Read the model definition and answer for the solid it produces. Units are mm, in the model's axes. A direction names the side the tool comes from. Round coordinates to 2 decimals unless told otherwise and drop trailing zeros. Order: outer loops, then holes, each group sorted by start corner. A loop starts at its lowest first (then second) coordinate and runs counter-clockwise, first axis right, second up.
Autodesk Inventor part; units mm, degrees
ref_plane "YZ Plane" through (0, 0, 0) normal (1, 0, 0) x (0, 1, 0)
ref_plane "XZ Plane" through (0, 0, 0) normal (0, 1, 0) x (-1, 0, 0)
ref_plane "XY Plane" through (0, 0, 0) normal (0, 0, 1) x (1, 0, 0)
sketch "Sketch1" plane through (0, 0, 0) normal (0, 1, 0) x (-1, 0, 0)
  line L0 (-30, -30) -> (30, -30)
  line L1 (30, -30) -> (30, 30)
  line L2 (30, 30) -> (-30, 30)
  line L3 (-30, 30) -> (-30, -30)
  line L4 (-30, -30) -> (30, 30) construction
  line L5 (30, -30) -> (-30, 30) construction
  circle A0 centre (0, 0) radius 7.5
  circle A1 centre (-25, 25) radius 1.95
  circle A2 centre (0, 25) radius 1.95
  circle A3 centre (0, 25) radius 1.95
  circle A4 centre (25, 0) radius 1.95
  circle A5 centre (25, -25) radius 1.95
  circle A6 centre (-25, 25) radius 1.95
  circle A7 centre (-25, -25) radius 1.95
  circle A8 centre (25, 25) radius 1.95
  circle A9 centre (-25, 0) radius 1.95
  circle A10 centre (0, -25) radius 1.95
  line L6 (28, 30) -> (30, 28)
  line L7 (30, 28) -> (30, -28)
  line L8 (30, -28) -> (28, -30)
  line L9 (28, -30) -> (-28, -30)
  line L10 (-28, -30) -> (-30, -28)
  line L11 (-30, -28) -> (-30, 28)
  line L12 (-30, 28) -> (-28, 30)
  line L13 (-28, 30) -> (28, 30)
  dimension "d0" = 60
  dimension "d1" = 60
  dimension "d13" = 15
extrude "Extrusion1" add sketch "Sketch1" along normal blind 12 contours L3 L10 L0 | L10 L3 L12 L2 L6 L1 L8 L0 | L8 L1 L0 | L3 L2 L12 | L6 L2 L1 | A1 | A2 | A4 | A5 | A7 | A8 | A9 | A10
sketch "Sketch2" plane through (0, 12, 0) normal (0, 1, 0) x (1, 0, 0)
  line L0 (30, 30) -> (-30, 30)
  line L1 (-30, 30) -> (-30, -30)
  line L2 (-30, -30) -> (30, -30)
  line L3 (30, -30) -> (30, 30)
  line L4 (17.5, -17.5) -> (-17.5, -17.5)
  line L5 (-17.5, -17.5) -> (-17.5, 17.5)
  line L6 (-17.5, 17.5) -> (17.5, 17.5)
  line L7 (17.5, 17.5) -> (17.5, -17.5)
  line L8 (17.5, -17.5) -> (-17.5, 17.5) construction
  line L9 (-17.5, -17.5) -> (17.5, 17.5) construction
  line L10 (0, -17.5) -> (0, 17.5)
  line L11 (-17.5, 0) -> (17.5, 0)
  point P0 (0, 0)
  dimension "d4" = 35
  dimension "d5" = 35
hole "Hole1" at (-17.5, 12, 17.5) at (-17.5, 12, -17.5) at (17.5, 12, -17.5) at (17.5, 12, 17.5) direction (0, -1, 0) diameter 3.9 depth 10 tip angle 118
chamfer "Chamfer1" distance 2 angle 45 4 edges at (30, 6, 30) (30, 6, -30) (-30, 6, -30) (-30, 6, 30)
sketch "Sketch3" plane through (0, 12, 0) normal (0, 1, 0) x (1, 0, 0)
  line L0 (-28, -30) -> (-30, -28)
  line L1 (-28, -30) -> (28, -30)
  line L2 (30, -28) -> (28, -30)
  line L3 (30, -28) -> (30, 28)
  line L4 (28, 30) -> (30, 28)
  line L5 (28, 30) -> (-28, 30)
  line L6 (-30, 28) -> (-28, 30)
  line L7 (-30, 28) -> (-30, -28)
  circle A0 centre (17.5, 17.5) radius 1.95
  circle A1 centre (-17.5, -17.5) radius 1.95
  circle A2 centre (-17.5, 17.5) radius 1.95
  circle A3 centre (17.5, -17.5) radius 1.95
  circle A4 centre (0, 0) radius 7.5
  line L8 (25, -25) -> (-25, -25)
  line L9 (-25, -25) -> (-25, 25)
  line L10 (-25, 25) -> (25, 25)
  line L11 (25, 25) -> (25, -25)
  line L12 (25, -25) -> (-25, 25) construction
  line L13 (-25, -25) -> (25, 25) construction
  dimension "d17" = 50
  dimension "d18" = 50
hole "Hole2" at (-25, 12, -25) at (25, 12, -25) at (25, 12, 25) at (-25, 12, 25) direction (0, -1, 0) diameter 4.65 end through all
sketch "Sketch4" plane through (30, 0, 28) normal (1, 0, 0) x (0, 0, -1)
  line L0 (56, 12) -> (56, 0)
  line L1 (0, 12) -> (56, 12)
  line L2 (0, 0) -> (0, 12)
  line L3 (0, 0) -> (56, 0)
  circle A0 centre (28, 8) radius 1.5
  line L4 (-2, 12) -> (-2, 0)
  point P0 (28, 0)
  dimension "d26" = 3
  dimension "d27" = 4
  dimension "d28" = 30
extrude "Extrusion2" cut sketch "Sketch4" against normal through all contours A0
sketch "Sketch5" plane through (0, 12, 0) normal (0, 1, 0) x (1, 0, 0)
  circle A0 centre (25, -25) radius 2.325
  circle A1 centre (-25, -25) radius 2.325
  circle A2 centre (25, 25) radius 2.325
  circle A3 centre (-25, 25) radius 2.325
  circle A4 centre (10, -25) radius 1.45
  circle A5 centre (-10, -25) radius 1.45
  circle A6 centre (10, 25) radius 1.45
  circle A7 centre (-10, 25) radius 1.45
  point P0 (0, 0)
  dimension "d31" = 2.9
  dimension "d32" = 2.9
  dimension "d33" = 15
  dimension "d34" = 15
  dimension "d35" = 2.9
  dimension "d36" = 2.9
extrude "Extrusion3" cut sketch "Sketch5" against normal blind 10 contours A4 | A5 | A6 | A7
pattern_circular "Circular Pattern1" count 2 over 90 about axis through (0, 0, 0) along (0, 1, 0) of "Extrusion3"
properties part number "00_XY_stage-CHUO_SEIKI_LD-647-R1-Top"
Q1. Flat-ended cylindrical pins translate along their axes: pin 1 (1.4 mm diameter, centred on x = -24.5, z = 10, fed in from +Y); pin 2 (3.5 mm diameter, centred on x = -25, z = -25, fed in from +Y); pin 3 (3 mm diameter, centred on x = 17.5, z = 17.5, fed in from +Y). Find the tip coordinate at first contact, or state that the pin passes through.
Outcome:
pin 1: stops at y = 2
pin 2: passes through
pin 3: stops at y = 1.73
Q2. For faces 3 (the face through (-22.73, 5.92, -25.5)), 4 (the face through (-11.15, 7.07, -24.12)), determine the directions among +Z, -Z, +X, -X, +Y, -Y from which every point of the face is accessible in a straight line to the end or side of a thin tool.
Outcome:
face 3: +Y, -Y
face 4: +Y
Q3. For a pull along Z with two mould halves and no side action, classify faces 1 (the face through (29, 6, 29)), 2 (the face through (-10, 2, 25)) as released by +Z, released by -Z, zero draft, split by the parting line, or undercut.
Outcome:
face 1: released by +Z
face 2: undercut
Q4. A cutting plane is placed at C-C, the plane x = 0. Give the vertices of the cut face in (y, z), plus the area to 3 significant figures.
Outcome:
outline: (0, -30) - (12, -30) - (12, -7.5) - (0, -7.5) - close; (0, 7.5) - (12, 7.5) - (12, 30) - (0, 30) - close
area: 540 mm2
Q5. A cutting plane is placed at A-A, the plane x = 25. Give the vertices of the cut face in (y, z) (3 decimals), plus the area to 3 significant figures.
Outcome:
outline: (0, -30) - (12, -30) - (12, -27.325) - (0, -27.325) - close; (0, -22.675) - (12, -22.675) - (12, -11.45) - (2, -11.45) - (2, -8.55) - (12, -8.55) - (12, 8.55) - (2, 8.55) - (2, 11.45) - (12, 11.45) - (12, 22.675) - (0, 22.675) - close; (0, 27.325) - (12, 27.325) - (12, 30) - (0, 30) - close; hole circle Ø3 at (8, 0)
area: 543 mm2
Q6. Straight lines are drawn through the part: probe 1 along X at (y, z) = (6.5, 25) (3 decimals); probe 2 along X at (y, z) = (4.5, -10). For each, find the intervals that lie inside material, in ascending order.
Outcome:
probe 1: x = -30 to -27.325, -22.675 to -11.45, -8.55 to 8.55, 11.45 to 22.675, 27.325 to 30
probe 2: x = -30 to -26.45, -23.55 to 23.55, 26.45 to 30
Q7. A cutting plane is placed at D-D, the plane z = 25. Give the vertices of the cut face in (x, y) (3 decimals), plus the area to 3 significant figures.
Outcome:
outline: (-30, 0) - (-27.325, 0) - (-27.325, 12) - (-30, 12) - close; (-22.675, 0) - (22.675, 0) - (22.675, 12) - (11.45, 12) - (11.45, 2) - (8.55, 2) - (8.55, 12) - (-8.55, 12) - (-8.55, 2) - (-11.45, 2) - (-11.45, 12) - (-22.675, 12) - close; (27.325, 0) - (30, 0) - (30, 12) - (27.325, 12) - close
area: 550 mm2
Q8. A cutting plane is placed at B-B, the plane y = 8. Give the number of separate pieces and of enclosed holes in the cut face, plus the area to 3 significant figures.
Outcome:
separate pieces: 2
enclosed holes: 16
area: 3,110 mm2
